Geometry check sheet. Reference: the model listing, model coordinates, mm. A direction names the side the tool comes from. Give positions to 0.01 mm unless a question says otherwise; leave off trailing zeros. Order: outer loops, then holes, each group sorted by start corner. A loop starts at its lowest first (then second) coordinate and runs counter-clockwise, first axis right, second up. Notation, with made-up numbers: M 21.25,54.25 L 26.25,54.25 A10 ccw 26.25,66.25 Z; hole C 84,27 d2. An arc over 180 degrees is marked long. Answer as CSV lines item,"result". Start each with the question number.
Q1. Mould release check, pull along Y, two halves, no side actions. Record for faces 5 (the flat face through (11, -78, -40)), 6 (the flat face through (31, 24, -25)), 7 (the flat face through (8, -69, -27)): +Y half, -Y half, draft (parallel to the pull), parting line (faces both ways), or undercut.
Q2. Thickness scan on line 1 (Y direction, x = -17.5, z = 1.6); line 2 (Y direction, x = -33, z = -12.5); line 3 (Z direction, x = 2, y = -5). Record the ranges inside material, lowest first.
Q3. Section check C-C, the plane x = -1.5. Record the boundary of the cut face in (y, z), then the cut area to 3 significant figures.
Q4. Section check D-D, the plane y = 17.5. Record the boundary of the cut face in (x, z), then the cut area to 4 significant figures.
Q5. Section check B-B, the plane z = -12. Record the boundary of the cut face in (x, y).
Q6. Set-up check for faces 1 (the flat face through (28, -69, -16)), 2 (the flat face through (0, -48, 0)), 3 (the flat face through (-36, 29, -26)), 4 (the flat face through (-34, 37, -41)): record each of +Z, -Z, +X, -X, +Y, -Y from which the full face is reachable in a straight line by a thin tool's end or side.
Q7. Go/stop test with flat-tipped pins: pin 1 (2.5 mm diameter, centred on x = 22.5, y = 40, fed in from -Z); pin 2 (12 mm diameter, centred on y = -72, z = -20, fed in from -X); pin 3 (11 mm diameter, centred on x = 28, y = -72.5, fed in from +Z); pin 4 (3 mm diameter, centred on x = -31.5, z = -33, fed in from -Y). Record where each tip stops, or that it passes through.
Q8. Section check A-A, the plane y = 40. Record the boundary of the cut face in (x, z).
```python
from build123d import *

# Parameters (mm, degrees)
SKETCH2_W           = 65
SKETCH2_H           = 90
SKETCH2_R           = 1.5
BOSS_EXTRUDE1_DEPTH = 5
SKETCH3_W           = 65
SKETCH3_H           = 5
BOSS_EXTRUDE2_DEPTH = 50
SKETCH4_W           = 23
SKETCH4_H           = 47
BOSS_EXTRUDE3_DEPTH = 1
SKETCH5_W           = 13
SKETCH5_H           = 35
BOSS_EXTRUDE4_DEPTH = 15
SKETCH6_W           = 60
SKETCH6_H           = 50
BOSS_EXTRUDE5_DEPTH = 75
SKETCH7_W           = 63
SKETCH7_H           = 60
BOSS_EXTRUDE6_DEPTH = 10
BOSS_EXTRUDE7_DEPTH = 17


with BuildPart() as part:
    # Sketch2 → Boss-Extrude1 (new body)
    with BuildSketch(Plane.XY):
        Rectangle(SKETCH2_W, SKETCH2_H)
        with Locations((-17.5, 40)):
            Circle(SKETCH2_R, mode=Mode.SUBTRACT)
        with Locations((22.5, 40)):
            Circle(SKETCH2_R, mode=Mode.SUBTRACT)
    extrude(amount=BOSS_EXTRUDE1_DEPTH)

    # Sketch3 → Boss-Extrude2 (add)
    with BuildSketch(Plane(origin=(0, 0, 0), x_dir=(-1, 0, 0), z_dir=(0, 0, -1))):
        with Locations((0, 26.5)):
            Rectangle(SKETCH3_W, SKETCH3_H)
    extrude(amount=BOSS_EXTRUDE2_DEPTH)

    # Sketch4 → Boss-Extrude3 (add)
    with BuildSketch(Plane(origin=(0, 29, 0), x_dir=(1, 0, 0), z_dir=(0, 1, 0))):
        with Locations((-28.787234074, 25.5)):
            Rectangle(SKETCH4_W, SKETCH4_H)
    extrude(amount=BOSS_EXTRUDE3_DEPTH)

    # Sketch5 → Boss-Extrude4 (add)
    with BuildSketch(Plane(origin=(0, 30, 0), x_dir=(1, 0, 0), z_dir=(0, 1, 0))):
        with Locations((-33.787234074, 23.5)):
            Rectangle(SKETCH5_W, SKETCH5_H)
    extrude(amount=BOSS_EXTRUDE4_DEPTH)

    # Sketch6 → Boss-Extrude5 (add)
    with BuildSketch(Plane.XZ.offset(-24)):
        with Locations((0, -25)):
            Rectangle(SKETCH6_W, SKETCH6_H)
    extrude(amount=BOSS_EXTRUDE5_DEPTH)

    # Sketch7 → Boss-Extrude6 (add)
    with BuildSketch(Plane.XZ.offset(51)):
        with Locations((1, -25)):
            Rectangle(SKETCH7_W, SKETCH7_H)
    extrude(amount=BOSS_EXTRUDE6_DEPTH)

    # Sketch8 → Boss-Extrude7 (add)
    with BuildSketch(Plane.XZ.offset(61)):
        Polygon((-7.5, -45), (22.5, -45), (22.5, -41), (22.5, -27), (-7.5, -27), align=None)
        Polygon((22.5, -55), (22.5, -45), (-7.5, -45), (-22.5, -45), (-22.5, -55), align=None)
        Polygon((22.5, -27), (22.5, -41), (32.5, -41), (32.5, -16), (22.5, -16), align=None)
    extrude(amount=BOSS_EXTRUDE7_DEPTH)


solid = part.part
```
Answer block:
1,face 5,"-Y half"
1,face 6,"undercut"
1,face 7,"draft"
2,line 1,"y = -61 to -51, -45 to 38.5, 41.5 to 45"
2,line 2,"y = 29 to 45"
2,line 3,"z = -50 to 5"
3,outline,"M -78,-55 L -51,-55 L -51,-50 L 29,-50 L 29,0 L 45,0 L 45,5 L -45,5 L -45,0 L -51,0 L -51,5 L -61,5 L -61,-27 L -78,-27 Z"
3,area,"5,530 mm2"
4,outline,"M -32.5,0 L -30,0 L -30,-50 L 30,-50 L 30,0 L 32.5,0 L 32.5,5 L -32.5,5 Z"
4,area,"3,325 mm2"
5,outline,"M -40.29,29 L -32.5,29 L -32.5,24 L -30,24 L -30,-51 L -30.5,-51 L -30.5,-61 L 32.5,-61 L 32.5,-51 L 30,-51 L 30,24 L 32.5,24 L 32.5,29 L -17.29,29 L -17.29,30 L -27.29,30 L -27.29,45 L -40.29,45 Z"
6,face 1,"+Z, +X, -X, -Y"
6,face 2,"+Z, +X, -X"
6,face 3,"+Z, -Z, -X, -Y"
6,face 4,"-Z, +X, -X, +Y"
7,pin 1,"passes through"
7,pin 2,"stops at x = 22.5"
7,pin 3,"stops at z = -16"
7,pin 4,"stops at y = -61"
8,outline,"M -40.29,-41 L -27.29,-41 L -27.29,-6 L -40.29,-6 Z; M -32.5,0 L -19,0 L -19,5 L -32.5,5 Z; M -16,0 L 21,0 L 21,5 L -16,5 Z; M 24,0 L 32.5,0 L 32.5,5 L 24,5 Z"
